Part print with two shaded views. Sizes in mm from the minimum x, y, z corner. Round coordinates to 2 decimals unless told otherwise and drop trailing zeros. Order: outer loops, then holes, each group sorted by start corner. A loop starts at its lowest first (then second) coordinate and runs counter-clockwise, first axis right, second up. Notation, with made-up numbers: (42, 27.25) -> (65, 27.25) arc R14 cw to (65, 36.25) -> close; hole circle Ø4 at (-4.75, 73.5). An arc over 180 degrees is marked (long way). Use a Markdown table: item, result. Add a question column.
Item 1: Pin check, flat tips, straight feed: pin 1 (12 mm diameter, centred on y = 28, z = 75.5, fed in from +X); pin 2 (13 mm diameter, centred on x = 72.7, z = 22.7, fed in from +Y); pin 3 (3 mm diameter, centred on y = 9, z = 28.5, fed in from +X); pin 4 (1 mm diameter, centred on x = 124.5, y = 23, fed in from +Z). Stop position of each tip, or through.
Item 2: Slice it at D-D, the plane x = 131. Give the cut face in (y, z), plus the area to 3 significant figures.
Item 3: Slice it at C-C, the plane y = 2. Give the cut face in (x, z), plus the area to 3 significant figures.
Item 4: Slice it at B-B, the plane z = 97.7. Give the cut face in (x, y).
Item 5: Probe L1, parallel to X at y = 23, z = 97.7; L2, parallel to X at y = 15, z = 97; L3, parallel to X at y = 18, z = 22 (1 decimal). List the from-to ranges inside material, lowest first.
Item 6: Slice it at A-A, the plane z = 72.7. Give the cut face in (x, y).
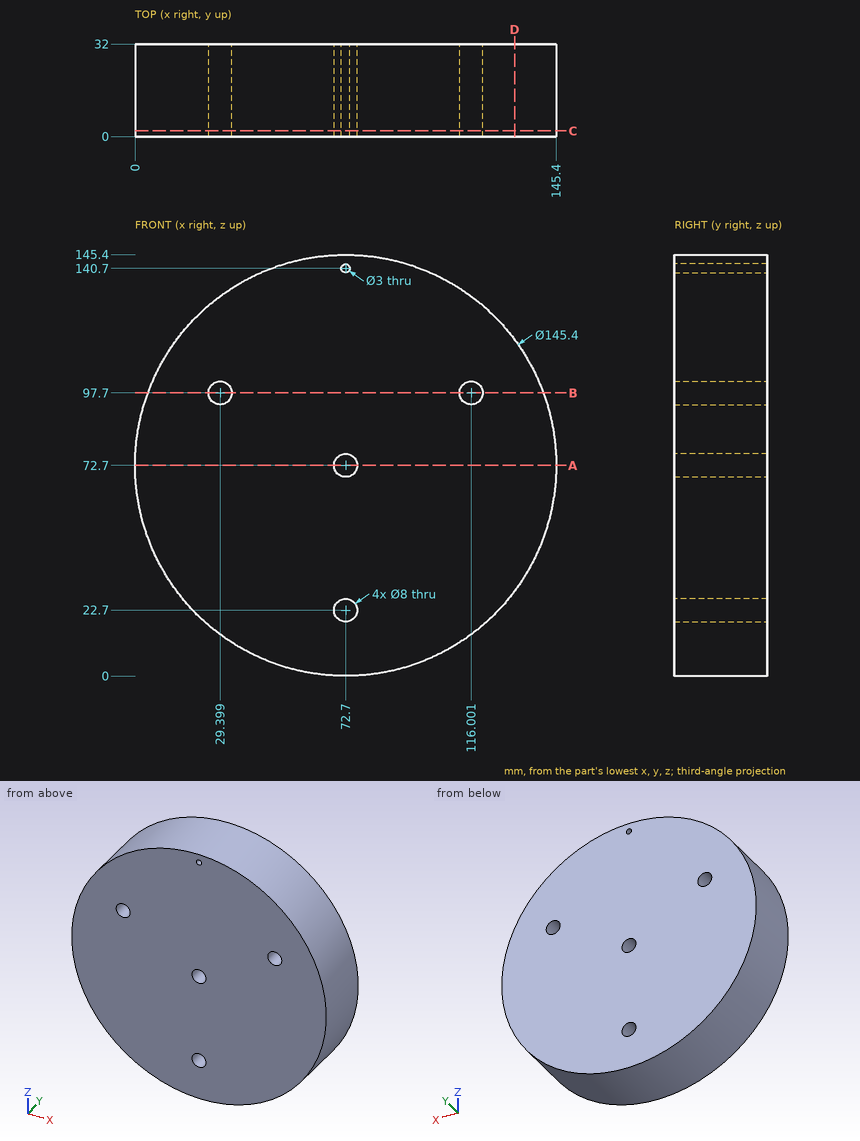
Check sheet entries:
| question | item | result |
|---|---|---|
| 1 | pin 1 | x = 145.4 |
| 1 | pin 2 | y = 32 |
| 1 | pin 3 | x = 131.54 |
| 1 | pin 4 | z = 124.21 |
| 2 | outline | (0, 29.27) -> (32, 29.27) -> (32, 116.13) -> (0, 116.13) -> close |
| 2 | area | 2,780 mm2 |
| 3 | outline | circle Ø145.4 at (72.7, 72.7); hole circle Ø8 at (29.4, 97.7); hole circle Ø8 at (72.7, 22.7); hole circle Ø8 at (72.7, 72.7); hole circle Ø3 at (72.7, 140.7); hole circle Ø8 at (116, 97.7) |
| 3 | area | 16,400 mm2 |
| 4 | outline | (4.43, 0) -> (25.4, 0) -> (25.4, 32) -> (4.43, 32) -> close; (33.4, 0) -> (112, 0) -> (112, 32) -> (33.4, 32) -> close; (120, 0) -> (140.97, 0) -> (140.97, 32) -> (120, 32) -> close |
| 5 | L1 | 4.43 to 25.4, 33.4 to 112, 120 to 140.97 |
| 5 | L2 | 4.18 to 25.46, 33.34 to 112.06, 119.94 to 141.22 |
| 5 | L3 | 20.6 to 68.8, 76.6 to 124.8 |
| 6 | outline | (0, 0) -> (68.7, 0) -> (68.7, 32) -> (0, 32) -> close; (76.7, 0) -> (145.4, 0) -> (145.4, 32) -> (76.7, 32) -> close |
